from build123d import *

# Parameters (mm, degrees)
BASPROSKE_W        = 13
BASPROSKE_H        = 10.5
TOOTHCUT_DEPTH     = 20.735754356
TEETHCUTS_COUNT    = 10
TEETHCUTS_ANGLE    = 324
BORSKE_R           = 1.5
BORE_DEPTH         = 50.0000508
CUT_EXTRUDE1_REACH = 21.504
SKETCH1_R          = 4.05
CHAMFER1_SIZE      = 0.5


with BuildPart() as part:
    # BasProSke → Base-Revolve (revolve)
    with BuildSketch(Plane(origin=(0, 0, 0), x_dir=(1, 0, 0), z_dir=(0, 1, 0)), mode=Mode.PRIVATE) as base_revolve_sk:
        with Locations((6.5, 5.25)):
            Rectangle(BASPROSKE_W, BASPROSKE_H)
    revolve(base_revolve_sk.sketch.rotate(Axis((-10, 0, 0), (1, 0, 0)), 180), axis=Axis((-10, 0, 0), (1, 0, 0)))

    # TooCutSke → ToothCut (cut, through all)
    with BuildSketch(Plane(origin=(0, 0, 0), x_dir=(0, 0, -1), z_dir=(1, 0, 0))):
        with BuildLine():
            ThreePointArc((1.019600066, 6.481797432), (0, 6.5615), (-1.019600066, 6.481797432))
            ThreePointArc((-1.019600066, 6.481797432), (-1.451036104, 8.608938557), (-3.053606956, 10.072712133))
            ThreePointArc((-3.053606956, 10.072712133), (0, 10.5254), (3.053606956, 10.072712133))
            ThreePointArc((3.053606956, 10.072712133), (1.451036104, 8.608938557), (1.019600066, 6.481797432))
        make_face()
    toothcut = extrude(amount=TOOTHCUT_DEPTH, mode=Mode.SUBTRACT)

    # TeethCuts: ToothCut ×10 about axis
    teethcuts_axis = Axis((-10, 0, 0), (1, 0, 0))
    for i in range(1, TEETHCUTS_COUNT):
        add(toothcut.rotate(teethcuts_axis, i * TEETHCUTS_ANGLE / (TEETHCUTS_COUNT - 1)), mode=Mode.SUBTRACT)

    # BorSke → Bore (cut, symmetric)
    with BuildSketch(Plane(origin=(0, 0, 0), x_dir=(0, 0, -1), z_dir=(1, 0, 0))):
        with Locations(Location((0, 0, 0), (0, 0, 180))):
            Circle(BORSKE_R)
    extrude(amount=BORE_DEPTH, both=True, mode=Mode.SUBTRACT)

    # Sketch1 → Cut-Extrude1 (cut, up to next)
    with BuildSketch(Plane.ZY, mode=Mode.PRIVATE) as cut_extrude1_sk1:
        Circle(SKETCH1_R)
    cut_extrude1_tool1 = extrude(cut_extrude1_sk1.sketch, amount=-CUT_EXTRUDE1_REACH, mode=Mode.PRIVATE) & part.part
    add(cut_extrude1_tool1.solids().sort_by_distance((0, 0, 0))[0], mode=Mode.SUBTRACT)

    # Chamfer1
    chamfer1_edges = [part.edges().sort_by_distance(p)[0] for p in [
        (0, 0, -4.05),
        (13, 0, -4.05),
    ]]
    chamfer(chamfer1_edges, length=CHAMFER1_SIZE)


solid = part.part
For this review, take the finished solid that the model builds, in its own axes (mm). Coordinates: 2 decimals unless noted, no trailing zeros. Loops run counter-clockwise (first coordinate to the right, second up) from the corner with the lowest first, then second, coordinate; pieces in that order, holes last. Notation, with made-up numbers: (-0.75, 82) -> (30.25, 82) arc R30 ccw to (30.25, 119) -> close; hole circle Ø3 at (14.5, -34.75). An arc over 180 degrees is marked (long way). Write each question's results on one line, items separated by ' | '.
Q1. To check wall thickness, follow line 1 along Y through (x, z) = (7.75, 0); line 2 along Z through (x, y) = (8.25, -2.25); line 3 along Y through (x, z) = (6.5, -5.75). State the ranges of each line that lie inside material, in increasing order. Write a range as [from, to].
Taken from the geometry:
line 1: [-6.56, -4.05], [4.05, 6.56] | line 2: [-6.16, -3.37], [3.37, 6.16] | line 3: [-5.84, 5.84]
Q2. Mouldability with a two-part tool opening along Y and no side actions: class faces 1 (the flat face through (13, -5, 0)), 2 (the cylindrical face through (6.41, -1.29, -8.59)) as +Y half, -Y half, draft (parallel to the pull), parting line (faces both ways), or undercut.
Taken from the geometry:
face 1: draft | face 2: undercut
Q3. Add section B-B, the plane y = -8.25. State the section outline as (x, z) points.
Taken from the geometry:
outline: (0, -3.91) -> (13, -3.91) -> (13, -1.27) -> (0, -1.27) -> close; (0, 1.27) -> (13, 1.27) -> (13, 3.91) -> (0, 3.91) -> close
Q4. Add section A-A, the plane z = 0. State the section outline as (x, y) points, then the cut area to 3 significant figures.
Taken from the geometry:
outline: (0, -6.56) -> (13, -6.56) -> (13, -4.55) -> (12.5, -4.05) -> (0.5, -4.05) -> (0, -4.55) -> close; (0, 4.55) -> (0.5, 4.05) -> (12.5, 4.05) -> (13, 4.55) -> (13, 6.56) -> (0, 6.56) -> close | area: 64.8 mm²
Q5. For pin 1 Ø3 at (x, z) = (3.5, -7.5) entering from +Y; pin 2 Ø2 at (x, y) = (2.5, -6.5) entering from +Z; pin 3 Ø6 at (x, z) = (4.5, -2) entering from +Y, all flat-tipped, find the tip position at first contact; note any pin that passes through.
Taken from the geometry:
pin 1: y = 6.43 | pin 2: z = 8.63 | pin 3: y = 10.06
Q6. Add section C-C, the plane z = -7.75. State the section outline as (x, y) points.
Taken from the geometry:
outline: (0, -6.43) -> (13, -6.43) -> (13, -4.05) -> (0, -4.05) -> close; (0, -1.35) -> (13, -1.35) -> (13, 1.35) -> (0, 1.35) -> close; (0, 4.05) -> (13, 4.05) -> (13, 6.43) -> (0, 6.43) -> close
